The listing builds one solid part. Answer for the finished solid, in the listing's coordinates (mm). Face numbers are marked on the shaded views. A direction names the side the tool comes from. Round coordinates to 2 decimals unless told otherwise and drop trailing zeros. Write each loop counter-clockwise with the first axis right and the second up, starting at its lowest first coordinate (ties: lowest second). Pieces come first, ordered by that corner, then holes. Notation, with made-up numbers: M 71,-39.5 L 99,-39.5 A24 ccw 99,-12.5 Z; hole C 49,-27 d3. An arc over 180 degrees is marked long. One line per item, written item: value. Start each with the question number.
(1) Section B-B (y = 0) is taken. Determine the outline of the cut face in (x, z).
(2) Section C-C (x = 0) is taken. Determine the outline of the cut face in (y, z).
(3) Section A-A (z = -163.5) is taken. Determine the outline of the cut face in (x, y).
(4) Consider probe 1 along X at (y, z) = (45.5, -140); probe 2 along Z at (x, y) = (144.5, 93); probe 3 along Z at (x, y) = (-37.5, 31.5). Determine where each line is inside the solid, lowest interval first.
(5) For the marked faces 1, 2 and 3, determine the directions among +Z, -Z, +X, -X, +Y, -Y from which every point of the face is accessible in a straight line to the end or side of a thin tool.
(6) For a pull along X with two mould halves and no side action, classify the marked faces 4, 5 and 6 as released by +X, released by -X, zero draft, split by the parting line, or undercut.
(7) Given P1, Ø4, axis at x = -132.5, y = 11.5, coming from the -Z side; P2, Ø4, axis at x = 13.5, y = -79, coming from the +Z side, each flat-ended and moving along its own axis, determine where each tip first touches the part or whether it passes through.
(8) Section D-D (z = -422) is taken. Determine the outline of the cut face in (x, y).
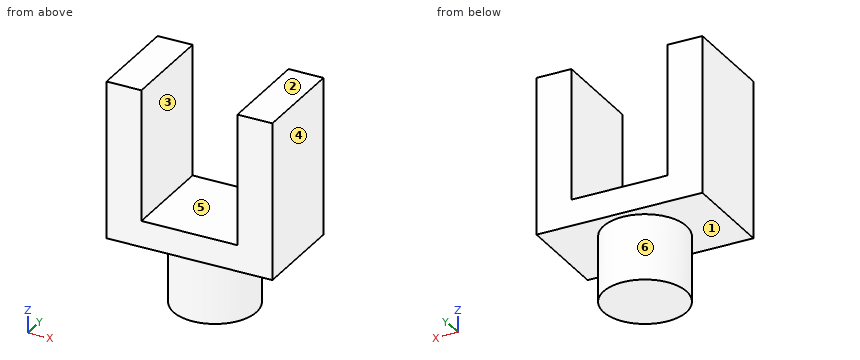
Autodesk Inventor part; units mm, degrees
ref_plane "YZ Plane" through (0, 0, 0) normal (1, 0, 0) x (0, 1, 0)
ref_plane "XZ Plane" through (0, 0, 0) normal (0, 1, 0) x (-1, 0, 0)
ref_plane "XY Plane" through (0, 0, 0) normal (0, 0, 1) x (1, 0, 0)
sketch "Sketch1" plane through (0, 0, 0) normal (0, 0, 1) x (1, 0, 0)
  line L0 (-190, 110) -> (-110, 110)
  line L1 (-110, 110) -> (-110, -110)
  line L2 (-110, -110) -> (-190, -110)
  line L3 (-190, -110) -> (-190, 110)
  line L4 (-190, 110) -> (-110, -110) construction
  line L5 (-110, 110) -> (-190, -110) construction
  line L6 (0, 0) -> (0, 2) construction
  line L7 (190, 110) -> (110, 110)
  line L8 (110, 110) -> (110, -110)
  line L9 (110, -110) -> (190, -110)
  line L10 (190, -110) -> (190, 110)
  line L11 (190, 110) -> (110, -110) construction
  line L12 (110, 110) -> (190, -110) construction
  point P0 (-150, 0)
  point P1 (-150, 0)
  point P2 (150, 0)
  point P3 (150, 0)
  dimension "d1" = 150
  dimension "d2" = 80
  dimension "d3" = 220
  dimension "d4" = 2
extrude "Extrusion1" add sketch "Sketch1" against normal blind 300
sketch "Sketch2" plane through (0, 0, -300) normal (0, 0, -1) x (-1, 0, 0)
  line L0 (-110, 110) -> (-190, 110)
  line L1 (110, -110) -> (190, -110)
  line L2 (-190, 110) -> (190, 110)
  line L3 (190, 110) -> (190, -110)
  line L4 (190, -110) -> (-190, -110)
  line L5 (-190, -110) -> (-190, 110)
  point P0 (0, 0)
extrude "Extrusion2" add sketch "Sketch2" along normal blind 60
sketch "Sketch3" plane through (0, 0, -360) normal (0, 0, -1) x (-1, 0, 0)
  circle A0 centre (0, 0) radius 95
  dimension "d9" = 190
extrude "Extrusion3" add sketch "Sketch3" along normal blind 150
thread "Thread1"
equation "\"BendRadius\" = Thickness"
equation "\"BendReliefWidth\" = Thickness"
equation "\"BendReliefDepth\" = 0.5 * Thickness"
equation "\"CornerReliefSize\" = 4 * Thickness"
equation "\"MinimumRemnant\" = 2 * Thickness"
equation "\"TransitionRadius\" = BendRadius"
equation "\"JacobiRadiusSize\" = BendRadius"
equation "\"GapSize\" = Thickness"
properties part number "08_Gripper"
Recorded:
1. outline: M -190,-360 L -95,-360 L -95,-510 L 95,-510 L 95,-360 L 190,-360 L 190,0 L 110,0 L 110,-300 L -110,-300 L -110,0 L -190,0 Z
2. outline: M -110,-360 L -95,-360 L -95,-510 L 95,-510 L 95,-360 L 110,-360 L 110,-300 L -110,-300 Z
3. outline: M -190,-110 L -110,-110 L -110,110 L -190,110 Z; M 110,-110 L 190,-110 L 190,110 L 110,110 Z
4. probe 1: x = -190 to -110, 110 to 190
4. probe 2: z = -360 to 0
4. probe 3: z = -510 to -300
5. face 1: -Z
5. face 2: +Z, +X, -X, +Y, -Y
5. face 3: +Z, +Y, -Y
6. face 4: released by +X
6. face 5: undercut
6. face 6: split by the parting line
7. P1: stops at z = -360
7. P2: stops at z = -300
8. outline: C 0,0 d190
